Geometry check sheet. Reference: the model listing, model coordinates, mm. Round coordinates to 2 decimals unless told otherwise and drop trailing zeros. Write each loop counter-clockwise with the first axis right and the second up, starting at its lowest first coordinate (ties: lowest second). Pieces come first, ordered by that corner, then holes.
from build123d import *

# Parameters (mm, degrees)
F0_W     = 150
F0_H     = 100
F1_DEPTH = 3


with BuildPart() as f1:
    # F0 (on Front) → F1 (new body)
    with BuildSketch(Plane.XZ):
        with BuildLine():
            Line((243.11273, 314.536521), (-356.88727, 314.536521))
            ThreePointArc((-356.88727, 314.536521), (-371.029405, 308.678657), (-376.88727, 294.536521))
            Line((-376.88727, 294.536521), (-376.88727, -215.463479))
            Line((-376.88727, -215.463479), (-296.88727, -215.463479))
            ThreePointArc((-296.88727, -215.463479), (-56.88727, 24.536521), (183.11273, -215.463479))
            Line((183.11273, -215.463479), (263.11273, -215.463479))
            Line((263.11273, -215.463479), (263.11273, 294.536521))
            ThreePointArc((263.11273, 294.536521), (257.254866, 308.678657), (243.11273, 314.536521))
        make_face()
        with Locations((128.11273, 214.536521)):
            Rectangle(F0_W, F0_H, mode=Mode.SUBTRACT)
    extrude(amount=F1_DEPTH)


solid = f1.part
1. Release check for a two-part mould opening along X. For faces 1 (the face through (-62.16, -1.48, 24.48)), 2 (the face through (-61, -3, 112)), 3 (the face through (257.41, -1.48, 308.52)) record: +X half, -X half, draft (parallel to the pull), parting line (faces both ways), or undercut.
2. Section check B-B (y = -2.5). Record the cut outline in (x, z), plus the area to 3 significant figures.
3. Section check C-C (z = -97). Record the cut outline in (x, y).
4. Section check A-A (z = 228.5). Record the cut outline in (x, y).
5. Depth check by flat-ended pin: pin 1 Ø0.9 at (x, y) = (103, -1) entering from -Z. Enter the tip coordinate at first touch or a pass-through.
6. Scan lines: line 1 along X through (y, z) = (-1.05, 169); line 2 along Z through (x, y) = (183.5, -2.5); line 3 along Z through (x, y) = (87, -1.95). Record each from-to range of solid material in increasing order.
7. Section check D-D (x = -113). Record the cut outline in (y, z), plus the area to 3 significant figures.
Results below:
1. face 1: undercut
1. face 2: draft
1. face 3: +X half
2. outline: (-376.89, -215.46) - (-296.89, -215.46) arc R240 cw to (183.11, -215.46) - (263.11, -215.46) - (263.11, 294.54) arc R20 ccw to (243.11, 314.54) - (-356.89, 314.54) arc R20 ccw to (-376.89, 294.54) - close; hole (53.11, 164.54) - (203.11, 164.54) - (203.11, 264.54) - (53.11, 264.54) - close
2. area: 234,000 mm2
3. outline: (-376.89, -3) - (-265.61, -3) - (-265.61, 0) - (-376.89, 0) - close; (151.84, -3) - (263.11, -3) - (263.11, 0) - (151.84, 0) - close
4. outline: (-376.89, -3) - (53.11, -3) - (53.11, 0) - (-376.89, 0) - close; (203.11, -3) - (263.11, -3) - (263.11, 0) - (203.11, 0) - close
5. pin 1: stops at z = -36.88
6. line 1: x = -376.89 to 53.11, 203.11 to 263.11
6. line 2: z = -215.46 to 164.54, 264.54 to 314.54
6. line 3: z = -23.38 to 164.54, 264.54 to 314.54
7. outline: (-3, 17.88) - (0, 17.88) - (0, 314.54) - (-3, 314.54) - close
7. area: 890 mm2
